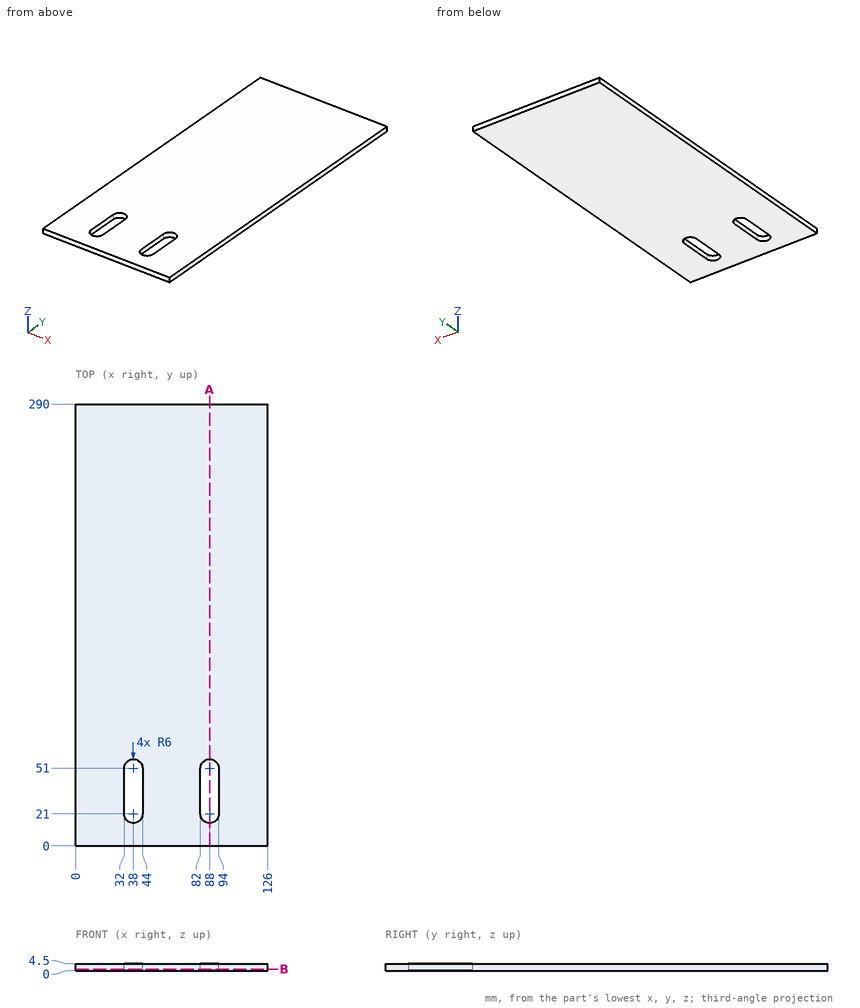
The figure shows three views and two pictorial views of one solid part (mm, origin at its lowest corner). Answer the questions. Round coordinates to 2 decimals unless told otherwise and drop trailing zeros. Write each loop counter-clockwise with the first axis right and the second up, starting at its lowest first coordinate (ties: lowest second). Pieces come first, ordered by that corner, then holes. Notation, with made-up numbers: (41, 5) -> (91, 5) arc R4 ccw to (91, 10) -> close; hole circle Ø3 at (59.5, 79.5). An arc over 180 degrees is marked (long way). Answer as a JSON object with one key per item and string values. Group by question number.
Q1. Section B-B (z = 1.1) is taken. Write down the section's boundary in (x, y).
Q2. Section A-A (x = 88) is taken. Write down the section's boundary in (y, z), plus the area to 3 significant figures.
Q3. Straight lines are drawn through the part: line 1 along X through (y, z) = (34, 2.45); line 2 along Y through (x, z) = (87.5, 3.2); line 3 along Y through (x, z) = (91.5, 1.95). For each, find the intervals that lie inside material, in ascending order.
Check values:
{
 "1": {"outline": "(0, 0) -> (126, 0) -> (126, 290) -> (0, 290) -> close; hole (32, 21) arc R6 ccw to (44, 21) -> (44, 51) arc R6 ccw to (32, 51) -> close; hole (82, 21) arc R6 ccw to (94, 21) -> (94, 51) arc R6 ccw to (82, 51) -> close"},
 "2": {"outline": "(0, 0) -> (15, 0) -> (15, 4.5) -> (0, 4.5) -> close; (57, 0) -> (290, 0) -> (290, 4.5) -> (57, 4.5) -> close", "area": "1,120 mm^2"},
 "3": {"line 1": "0 to 32, 44 to 82, 94 to 126", "line 2": "0 to 15.02, 56.98 to 290", "line 3": "0 to 16.13, 55.87 to 290"}
}
